```python
from build123d import *

# Parameters (mm, degrees)
SKETCH2_W           = 50
SKETCH2_H           = 55
SKETCH2_R           = 1.65
BOSS_EXTRUDE2_DEPTH = 6
CUT_EXTRUDE1_START  = 1.8
CUT_EXTRUDE1_DEPTH  = 2.4
SKETCH4_R           = 3
SKETCH4_R_2         = 1.65
BOSS_EXTRUDE3_DEPTH = 3.5
SKETCH5_R           = 3
CUT_EXTRUDE2_DEPTH  = 3
SKETCH6_W           = 50
SKETCH6_H           = 3.75
SKETCH6_H_2         = 6
CUT_EXTRUDE3_DEPTH  = 10


with BuildPart() as part:
    # Sketch2 → Boss-Extrude2 (new body)
    with BuildSketch(Plane(origin=(0, 0, 0), x_dir=(1, 0, 0), z_dir=(0, 1, 0))):
        with Locations((25, 27.5)):
            Rectangle(SKETCH2_W, SKETCH2_H)
        with Locations((6, 10)):
            Circle(SKETCH2_R, mode=Mode.SUBTRACT)
        with Locations((44, 10)):
            Circle(SKETCH2_R, mode=Mode.SUBTRACT)
        with Locations((44, 48)):
            Circle(SKETCH2_R, mode=Mode.SUBTRACT)
        with Locations((6, 48)):
            Circle(SKETCH2_R, mode=Mode.SUBTRACT)
        with Locations((6, 29)):
            Circle(SKETCH2_R, mode=Mode.SUBTRACT)
        with Locations((44, 29)):
            Circle(SKETCH2_R, mode=Mode.SUBTRACT)
    extrude(amount=BOSS_EXTRUDE2_DEPTH)

    # Sketch3 → Cut-Extrude1 (cut)
    with BuildSketch(Plane(origin=(0, 0, 0), x_dir=(1, 0, 0), z_dir=(0, 1, 0)).offset(CUT_EXTRUDE1_START)):
        Polygon((9.233161507, 48), (7.616580754, 50.8), (4.383419246, 50.8), (2.766838493, 48), (4.383419246, 45.2), (7.616580754, 45.2), align=None)
        Polygon((47.233161507, 48), (45.616580754, 50.8), (42.383419246, 50.8), (40.766838493, 48), (42.383419246, 45.2), (45.616580754, 45.2), align=None)
        Polygon((47.233161507, 10), (45.616580754, 12.8), (42.383419246, 12.8), (40.766838493, 10), (42.383419246, 7.2), (45.616580754, 7.2), align=None)
        Polygon((9.233161507, 10), (7.616580754, 12.8), (4.383419246, 12.8), (2.766838493, 10), (4.383419246, 7.2), (7.616580754, 7.2), align=None)
    extrude(amount=CUT_EXTRUDE1_DEPTH, mode=Mode.SUBTRACT)

    # Sketch4 → Boss-Extrude3 (add)
    with BuildSketch(Plane(origin=(0, 6, 0), x_dir=(1, 0, 0), z_dir=(0, 1, 0))):
        with Locations((6, 10)):
            Circle(SKETCH4_R)
        with Locations((6, 10)):
            Circle(SKETCH4_R_2, mode=Mode.SUBTRACT)
        with Locations((44, 10)):
            Circle(SKETCH4_R)
        with Locations((44, 10)):
            Circle(SKETCH4_R_2, mode=Mode.SUBTRACT)
        with Locations((6, 48)):
            Circle(SKETCH4_R)
        with Locations((6, 48)):
            Circle(SKETCH4_R_2, mode=Mode.SUBTRACT)
        with Locations((44, 48)):
            Circle(SKETCH4_R)
        with Locations((44, 48)):
            Circle(SKETCH4_R_2, mode=Mode.SUBTRACT)
    extrude(amount=BOSS_EXTRUDE3_DEPTH)

    # Sketch5 → Cut-Extrude2 (cut)
    with BuildSketch(Plane(origin=(0, 6, 0), x_dir=(1, 0, 0), z_dir=(0, 1, 0))):
        with Locations((6, 29)):
            Circle(SKETCH5_R)
        with Locations((44, 29)):
            Circle(SKETCH5_R)
    extrude(amount=-CUT_EXTRUDE2_DEPTH, mode=Mode.SUBTRACT)

    # Sketch6 → Cut-Extrude3 (cut)
    with BuildSketch(Plane(origin=(0, 6, 0), x_dir=(1, 0, 0), z_dir=(0, 1, 0))):
        with Locations((25, 53.125)):
            Rectangle(SKETCH6_W, SKETCH6_H)
        with Locations((25, 3)):
            Rectangle(SKETCH6_W, SKETCH6_H_2)
    extrude(amount=-CUT_EXTRUDE3_DEPTH, mode=Mode.SUBTRACT)


solid = part.part
```
Verification items for the finished model (mm, model axes). A direction names the side the tool comes from. Round coordinates to 2 decimals unless told otherwise and drop trailing zeros. Write each loop counter-clockwise with the first axis right and the second up, starting at its lowest first coordinate (ties: lowest second). Pieces come first, ordered by that corner, then holes. Notation, with made-up numbers: (53, 32) - (83, 32) arc R17 cw to (83, 43) - close; hole circle Ø10 at (-22.75, 6.5). An arc over 180 degrees is marked (long way). Answer as a JSON object with one key per item and string values. Group by question number.
Q1. Tool access check on faces 4 (the flat face through (6, 3, -7.2)), 5 (the cylindrical face through (41, 5, -29)), 6 (the flat face through (7.3, 9.5, -46.7)). Record the directions out of +Z, -Z, +X, -X, +Y, -Y that give a thin tool (end or side, any length) a straight path to the whole face; none if there is none.
Q2. Section check D-D, the plane x = 44. Give the number of separate pieces and of enclosed holes in the cut face, plus the area to 3 significant figures.
Q3. Section check B-B, the plane y = 8.75. Enter the section's corners in (x, z), plus the area to 3 significant figures.
Q4. Section check A-A, the plane z = -29. Enter the section's corners in (x, y).
Q5. Section check C-C, the plane y = 5. Enter the section's corners in (x, z), plus the area to 3 significant figures.
Q6. Thickness scan on line 1 (Z direction, x = 6, y = 7.75); line 2 (Z direction, x = 44, y = 0.6); line 3 (X direction, y = 4.75, z = -28.5). Record the ranges inside material, lowest first.
Q7. Go/stop test with flat-tipped pins: pin 1 Ø2.5 at (x, z) = (44, -10) entering from +Y; pin 2 Ø5.5 at (x, z) = (6, -29) entering from -Y; pin 3 Ø8 at (x, z) = (30, -31) entering from +Y. Record where each tip stops, or that it passes through.
Q8. Mould release check, pull along Y, two halves, no side actions. Record for faces 1 (the flat face through (46.436, 2.983, -49.38)), 2 (the flat face through (25, 0, -29)), 3 (the cylindrical face through (8.77, 4.52, -27.85)): released by +Y, released by -Y, zero draft, split by the parting line, or undercut.
Found:
{
 "1": {"face 4": "none", "face 5": "+Y", "face 6": "+Z, -Z, +X, -X, +Y"},
 "2": {"separate pieces": "4", "enclosed holes": "0", "area": "212 mm^2"},
 "3": {"outline": "circle Ø6 at (6, -48); circle Ø6 at (6, -10); circle Ø6 at (44, -48); circle Ø6 at (44, -10); hole circle Ø3.3 at (6, -48); hole circle Ø3.3 at (6, -10); hole circle Ø3.3 at (44, -48); hole circle Ø3.3 at (44, -10)", "area": "78.9 mm^2"},
 "4": {"outline": "(0, 0) - (4.35, 0) - (4.35, 3) - (3, 3) - (3, 6) - (0, 6) - close; (7.65, 0) - (42.35, 0) - (42.35, 3) - (41, 3) - (41, 6) - (9, 6) - (9, 3) - (7.65, 3) - close; (45.65, 0) - (50, 0) - (50, 6) - (47, 6) - (47, 3) - (45.65, 3) - close"},
 "5": {"outline": "(0, -51.25) - (50, -51.25) - (50, -6) - (0, -6) - close; hole circle Ø6 at (6, -29); hole circle Ø3.3 at (6, -48); hole circle Ø3.3 at (6, -10); hole circle Ø6 at (44, -29); hole circle Ø3.3 at (44, -48); hole circle Ø3.3 at (44, -10)", "area": "2,170 mm^2"},
 "6": {"line 1": "z = -51 to -49.65, -46.35 to -45, -13 to -11.65, -8.35 to -7", "line 2": "z = -51.25 to -49.65, -46.35 to -30.65, -27.35 to -11.65, -8.35 to -6", "line 3": "x = 0 to 3.04, 8.96 to 41.04, 46.96 to 50"},
 "7": {"pin 1": "passes through", "pin 2": "stops at y = 0", "pin 3": "stops at y = 6"},
 "8": {"face 1": "undercut", "face 2": "released by -Y", "face 3": "zero draft"}
}
